Could you check a few things on this drawing? It's one solid part, dimensions in mm from its lowest x, y, z. Give positions to 0.01 mm unless a question says otherwise; leave off trailing zeros. Loops run counter-clockwise (first coordinate to the right, second up) from the corner with the lowest first, then second, coordinate; pieces in that order, holes last. Notation, with made-up numbers: (15.25, 55.5) - (38.25, 55.5) arc R26 ccw to (38.25, 71.5) - close; hole circle Ø8 at (65.25, 83). An arc over 180 degrees is marked (long way). Write item = value, one per line.
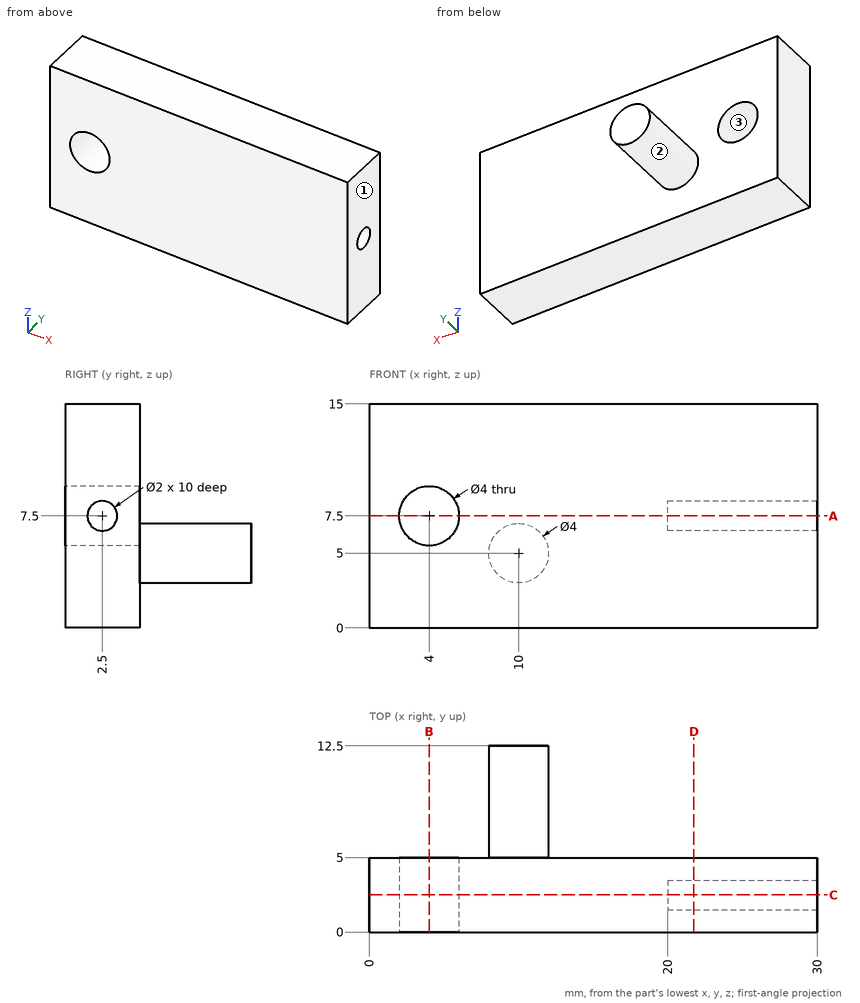
Q1. For pin 1 (1.5 mm diameter, centred on y = 9.5, z = 9, fed in from -X); pin 2 (5 mm diameter, centred on x = 10, y = 11, fed in from -Z); pin 3 (5 mm diameter, centred on x = 20, z = 4.5, fed in from +Y), each with a flat end and sliding along its axis, tell me the tip position at first contact or that it passes through.
Output:
pin_1 = through
pin_2 = 3
pin_3 = 5
Q2. Imagine slicing it at D-D, the plane x = 21.75. Write out the boundary of the cut face in (y, z), then the cut area to 3 significant figures.
Output:
outline = (0, 0) - (5, 0) - (5, 15) - (0, 15) - close; hole circle Ø2 at (2.5, 7.5)
area = 71.9 mm2
Q3. I need wall thicknesses on L1, parallel to X at y = 2.9, z = 7.5; L2, parallel to Y at x = 18.25, z = 7.75; L3, parallel to X at y = 4, z = 8.75. Which ranges of each line are inside material? Lowest first, please.
Output:
L1 = 0 to 2, 6 to 20
L2 = 0 to 5
L3 = 0 to 2.44, 5.56 to 30
Q4. Imagine slicing it at C-C, the plane y = 2.5. Write out the boundary of the cut face in (x, z).
Output:
outline = (0, 0) - (30, 0) - (30, 6.5) - (20, 6.5) - (20, 8.5) - (30, 8.5) - (30, 15) - (0, 15) - close; hole circle Ø4 at (4, 7.5)
Q5. Imagine slicing it at B-B, the plane x = 4. Write out the boundary of the cut face in (y, z), then the cut area to 3 significant figures.
Output:
outline = (0, 0) - (5, 0) - (5, 5.5) - (0, 5.5) - close; (0, 9.5) - (5, 9.5) - (5, 15) - (0, 15) - close
area = 55.0 mm2
Q6. Imagine slicing it at A-A, the plane z = 7.5. Write out the boundary of the cut face in (x, y), then the cut area to 3 significant figures.
Output:
outline = (0, 0) - (2, 0) - (2, 5) - (0, 5) - close; (6, 0) - (30, 0) - (30, 1.5) - (20, 1.5) - (20, 3.5) - (30, 3.5) - (30, 5) - (6, 5) - close
area = 110 mm2
Q7. We'd pull the mould along Z, two halves only. Please class the marked faces 1, 2 and 3: released by +Z, released by -Z, zero draft, split by the parting line, or undercut.
Output:
face_1 = zero draft
face_2 = split by the parting line
face_3 = undercut
